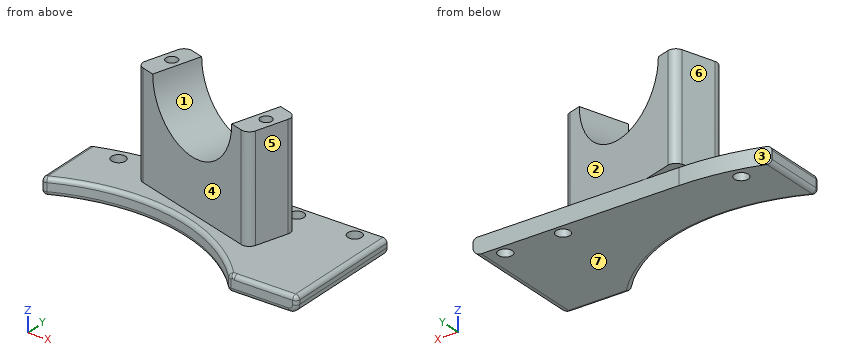
```python
from build123d import *

# Parameters (mm, degrees)
PAD_DEPTH       = 4
PAD001_DEPTH    = 25.5
SKETCH002_R     = 12.9
POCKET_DEPTH    = 36.8669197108
FILLET_R        = 2
FILLET001_R     = 1
FILLET002_R     = 1
FILLET003_R     = 1
SKETCH003_R     = 1.4
POCKET001_DEPTH = 12
SKETCH004_R     = 1.7
POCKET002_DEPTH = 4.0010001
FILLET004_R     = 2
FILLET005_R     = 1


with BuildPart() as part:
    # Sketch → Pad (new body)
    with BuildSketch(Plane.XY):
        with BuildLine():
            Line((33.5410196625, 30), (50, 30))
            Line((50, 30), (50, 60))
            Line((0, 60), (50, 60))
            ThreePointArc((0, 60), (-10.1461187235, 59.1359135792), (-20, 56.5685424949))
            Line((-20, 40.3112887415), (-20, 56.5685424949))
            ThreePointArc((33.5410196625, 30), (8.5100218715, 44.1880020792), (-20, 40.3112887415))
        make_face()
    extrude(amount=PAD_DEPTH)

    # Sketch001 → Pad001 (new body)
    with BuildSketch(Plane.XY.offset(4)):
        Polygon((-0.671183324, 62.6409760428), (33.7557878907, 52.1155946728), (30.247327434, 40.6399376012), (-4.1796437807, 51.1653189712), align=None)
    extrude(amount=PAD001_DEPTH)

    # Sketch002 → Pocket (cut, through all)
    with BuildSketch(Plane(origin=(17.4568210696, 57.098688906, 0), x_dir=(-0.956304756, 0.2923717047, 0), z_dir=(0.2923717047, 0.956304756, 0))):
        with Locations((0.956304756, 29.5)):
            Circle(SKETCH002_R)
    extrude(amount=-POCKET_DEPTH, mode=Mode.SUBTRACT)

    # Fillet
    fillet_edges = [part.edges().sort_by_distance(p)[0] for p in [
        (50, 45, 0),
    ]]
    fillet(fillet_edges, radius=FILLET_R)

    # Fillet001
    fillet001_edges = [part.edges().sort_by_distance(p)[0] for p in [
        (-20, 48.439916, 4),
    ]]
    fillet(fillet001_edges, radius=FILLET001_R)

    # Fillet002
    fillet002_edges = [part.edges().sort_by_distance(p)[0] for p in [
        (9.054169, 44.079724, 4),
    ]]
    fillet(fillet002_edges, radius=FILLET002_R)

    # Fillet003
    fillet003_edges = [part.edges().sort_by_distance(p)[0] for p in [
        (42.435596, 30, 4),
    ]]
    fillet(fillet003_edges, radius=FILLET003_R)

    # Sketch003 → Pocket001 (cut)
    with BuildSketch(Plane.XY.offset(29.5)):
        with Locations((0.2205096629, 56.6647829722)):
            Circle(SKETCH003_R)
        with Locations((29.6746961465, 47.6597344667)):
            Circle(SKETCH003_R)
    extrude(amount=-POCKET001_DEPTH, mode=Mode.SUBTRACT)

    # Sketch004 → Pocket002 (cut, through all)
    with BuildSketch(Plane.XY.offset(4)):
        with Locations((44, 57.5)):
            Circle(SKETCH004_R)
        with Locations((-12, 55.75)):
            Circle(SKETCH004_R)
        with Locations((30, 57.5)):
            Circle(SKETCH004_R)
    extrude(amount=-POCKET002_DEPTH, mode=Mode.SUBTRACT)

    # Fillet004
    fillet004_edges = [part.edges().sort_by_distance(p)[0] for p in [
        (-0.671183, 62.640976, 16.75),
        (33.755788, 52.115595, 16.75),
        (30.247327, 40.639938, 16.75),
        (-4.179644, 51.165319, 16.75),
    ]]
    fillet(fillet004_edges, radius=FILLET004_R)

    # Fillet005
    fillet005_edges = [part.edges().sort_by_distance(p)[0] for p in [
        (50, 45.5, 4),
    ]]
    fillet(fillet005_edges, radius=FILLET005_R)


solid = part.part
```
The model under review builds one solid part; all positions refer to its coordinate system, in mm. Face numbers are marked on the shaded views. A direction names the side the tool comes from. Give positions to 0.01 mm unless a question says otherwise; leave off trailing zeros. Write each loop counter-clockwise with the first axis right and the second up, starting at its lowest first coordinate (ties: lowest second). Pieces come first, ordered by that corner, then holes. Notation, with made-up numbers: M 87.25,79.5 L 124.25,79.5 A22 ccw 124.25,97.5 Z; hole C -25,-25 d10. An arc over 180 degrees is marked long. Write item = value, one per line. Start each with the question number.
Q1. Clearance check with flat-ended pins moving along their axes: pin 1 (10 mm diameter, centred on x = -3.5, z = 16, fed in from -Y); pin 2 (8.5 mm diameter, centred on x = 4, y = 42, fed in from +Z); pin 3 (0.6 mm diameter, centred on x = 1.5, y = 61.5, fed in from -Z); pin 4 (2 mm diameter, centred on x = -12, y = 55.75, fed in from +Z). State where each tip first meets the part, or that it passes through.
Q2. We need section B-B (x = 44). State the section outline as (y, z) points.
Q3. Mouldability with a two-part tool opening along X and no side actions: class the marked faces 1, 2 and 3 as released by +X, released by -X, zero draft, split by the parting line, or undercut.
Q4. We need section A-A (z = 26.25). State the section outline as (x, y) points, plus the area to 3 significant figures.
Q5. We need section C-C (z = 8.5). State the section outline as (x, y) points.
Q6. Machinability: for the marked faces 4, 5, 6 and 7, which of the approach directions +Z, -Z, +X, -X, +Y, -Y give a long, thin tool a straight path to every point of the face, cutting with its end or side? Answer none if there is none.
Q7. For line 1 (X direction, y = 55.5, z = 20.25); line 2 (Z direction, x = 42, y = 51); line 3 (Y direction, x = -12, z = 0.9), list the stretches that pass through material, from the lowest coordinate up.
Q8. We need section D-D (z = 22.5). State the section outline as (x, y) points.
Result set:
q1.pin_1 = 49.43
q1.pin_2 = 4
q1.pin_3 = 4
q1.pin_4 = through
q2.outline = M 30,1 A1 ccw 31,0 L 55.8,0 L 55.8,4 L 31,4 A1 ccw 30,3 Z; M 59.2,0 L 60,0 L 60,4 L 59.2,4 Z
q3.face_1 = undercut
q3.face_2 = released by +X
q3.face_3 = released by -X
q4.outline = M -3.59,53.08 A2 ccw -2.27,50.58 L 1.1,49.55 L 4.6,61.03 L 1.24,62.06 A2 ccw -1.26,60.73 Z; M 24.97,42.25 L 28.33,41.22 A2 ccw 30.83,42.55 L 33.17,50.2 A2 ccw 31.84,52.7 L 28.48,53.73 Z; hole C 0.22,56.66 d2.8; hole C 29.67,47.66 d2.8
q4.area = 117 mm2
q5.outline = M -3.59,53.08 A2 ccw -2.27,50.58 L 28.33,41.22 A2 ccw 30.83,42.55 L 33.17,50.2 A2 ccw 31.84,52.7 L 1.24,62.06 A2 ccw -1.26,60.73 Z
q6.face_4 = +Z, -X, -Y
q6.face_5 = +Z, +X, -Y
q6.face_6 = +Z, -X, +Y
q6.face_7 = -Z, +X, -X, +Y, -Y
q7.line_1 = -2.85 to -0.56, 1 to 6.57
q7.line_2 = 0 to 4
q7.line_3 = 43.38 to 54.05, 57.45 to 58.79
q8.outline = M -3.59,53.08 A2 ccw -2.27,50.58 L 2.67,49.07 L 6.18,60.55 L 1.24,62.06 A2 ccw -1.26,60.73 Z; M 23.4,42.73 L 28.33,41.22 A2 ccw 30.83,42.55 L 33.17,50.2 A2 ccw 31.84,52.7 L 26.9,54.21 Z; hole C 0.22,56.66 d2.8; hole C 29.67,47.66 d2.8
